```python
from build123d import *

# Parameters (mm, degrees)
BASEHEAD_DEPTH     = 4
SKETCH2_R          = 3
BASEBODY_DEPTH     = 25
SKETCH4_R          = 3.4
CUT_EXTRUDE1_DEPTH = 0.8
SKETCH6_R          = 0.8
HOLE_DEPTH         = 6
CIRPATTERN1_COUNT  = 2
CIRPATTERN1_ANGLE  = 60
LPATTERN10_COUNT   = 28
LPATTERN10_PITCH   = 0.6498


with BuildPart() as part:
    # Sketch1 → BaseHead (new body)
    with BuildSketch(Plane(origin=(0, 0, 0), x_dir=(0, 0, -1), z_dir=(1, 0, 0))):
        Polygon((5.773502692, 0), (2.886751346, 5), (-2.886751346, 5), (-5.773502692, 0), (-2.886751346, -5), (2.886751346, -5), align=None)
    extrude(amount=BASEHEAD_DEPTH)

    # Sketch2 → BaseBody (add)
    with BuildSketch(Plane(origin=(4, 0, 0), x_dir=(0, 0, -1), z_dir=(1, 0, 0))):
        Circle(SKETCH2_R)
    extrude(amount=BASEBODY_DEPTH)

    # Sketch3 → HeadChamfer (revolve, cut)
    with BuildSketch(Plane(origin=(3.161211974, 0, 2.612290718), x_dir=(0, 0, -1), z_dir=(0, 1, 0))):
        Polygon((8.38579341, 3.161211974), (8.38579341, 2.643099366), (6.962290718, 3.161211974), align=None)
    revolve(axis=Axis((-2.071354488, 0, 0), (1, 0, 0)), mode=Mode.SUBTRACT)

    # Sketch4 → Cut-Extrude1 (cut)
    with BuildSketch(Plane.ZY):
        Circle(SKETCH4_R)
    extrude(amount=-CUT_EXTRUDE1_DEPTH, mode=Mode.SUBTRACT)

    # Sketch5 → Cut-Revolve1 (revolve, cut)
    with BuildSketch(Plane(origin=(-2.92963122, 0, 7.92963122), x_dir=(0, 0, -1), z_dir=(0, 1, 0))):
        Polygon((10.92963122, -13.92963122), (10.60463122, -11.42963122), (10.60463122, -6.92963122), (13.27963122, -6.92963122), (13.27963122, -13.92963122), align=None)
    revolve(axis=Axis((-2.697175707, 0, 0), (1, 0, 0)), mode=Mode.SUBTRACT)

    # Sketch6 → Hole (cut, symmetric)
    with BuildSketch(Plane(origin=(0, 0, 0), x_dir=(1, 0, 0), z_dir=(0, 1, 0))):
        with Locations((2, 0)):
            Circle(SKETCH6_R)
    hole = extrude(amount=HOLE_DEPTH, both=True, mode=Mode.SUBTRACT)

    # CirPattern1: Hole ×2 about axis
    cirpattern1_axis = Axis((-2.697175707, 0, 0), (1, 0, 0))
    for i in range(1, CIRPATTERN1_COUNT):
        add(hole.rotate(cirpattern1_axis, i * CIRPATTERN1_ANGLE / (CIRPATTERN1_COUNT - 1)), mode=Mode.SUBTRACT)

    # Sketch7 → Cut-Revolve10 (revolve, cut)
    with BuildSketch(Plane.XY):
        Polygon((28.72925, 3.2), (29.27075, 3.2), (29.27075, 3), (29, 2.531047244), (28.72925, 3), align=None)
    cut_revolve10 = revolve(axis=Axis((28.86346516, 0, 0), (-1, 0, 0)), mode=Mode.SUBTRACT)

    # LPattern10: Cut-Revolve10 ×28
    with Locations(*[(-i * LPATTERN10_PITCH, 0, 0) for i in range(1, LPATTERN10_COUNT)]):
        add(cut_revolve10, mode=Mode.SUBTRACT)


solid = part.part
```
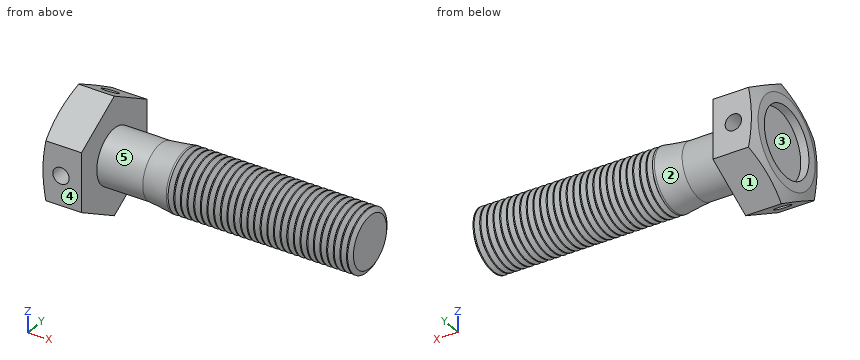
Part model, mm, in its own coordinate system. Face numbers are marked on the shaded views. A direction names the side the tool comes from. Give positions to 0.01 mm unless a question says otherwise; leave off trailing zeros. Order: outer loops, then holes, each group sorted by start corner. A loop starts at its lowest first (then second) coordinate and runs counter-clockwise, first axis right, second up. Notation, with made-up numbers: M 80,-14 L 110,-14 A21 cw 110,-4 Z; hole C 89.5,19 d8. An arc over 180 degrees is marked long. Use a Markdown table: item, result. Add a question column.
(1) Saw through at B-B, the plane x = 5. Give the cut face in (y, z) (3 decimals), and give its area (3 significant figures).
(2) Drop flat-ended pins along their axis: P1, Ø3.5, axis at y = 1, z = -1.5, coming from the -X side; P2, Ø3, axis at x = 16, y = -1, coming from the +Z side. Give the stop position or say it passes through.
(3) Probe line 1 along X through (y, z) = (2, 0); line 2 along Y through (x, z) = (0.6, 0); line 3 along X through (y, z) = (3, -2.25). List the from-to ranges inside material, lowest first. Write a range as [from, to].
(4) Saw through at A-A, the plane x = 2. Give the cut face in (y, z).
(5) Mould opens along Y. For the marked faces 3, 4 and 5 say: +Y half, -Y half, draft (parallel to the pull), parting line (faces both ways), or undercut.
(6) 3-axis set-ups, long thin cutter, end or side, ignore diameter. For the marked faces 1 and 2: which of +Z, -Z, +X, -X, +Y, -Y reach the whole face in a straight line?
Answer key:
| question | item | result |
|---|---|---|
| 1 | outline | C 0,0 d5.35 |
| 1 | area | 22.5 mm^2 |
| 2 | P1 | x = 0 |
| 2 | P2 | z = 3 |
| 3 | line 1 | [0.8, 1.2], [2.8, 29] |
| 3 | line 2 | [-5, -3.4], [3.4, 5] |
| 3 | line 3 | [0, 4] |
| 4 | outline | M -5,-2.89 L -3.19,-3.93 L -1.39,-0.8 L -5,-0.8 Z; M -5,0.8 L -0.46,0.8 L 1.81,4.73 L 0,5.77 L -5,2.89 Z; M -1.81,-4.73 L 0,-5.77 L 5,-2.89 L 5,-0.8 L 0.46,-0.8 Z; M 1.39,0.8 L 5,0.8 L 5,2.89 L 3.19,3.93 Z |
| 5 | face 3 | undercut |
| 5 | face 4 | -Y half |
| 5 | face 5 | parting line |
| 6 | face 1 | -Z, +X, -X, +Y |
| 6 | face 2 | none |
